Model file for the job. Use its own axes, mm. A direction names the side the tool comes from. Round coordinates to 2 decimals unless told otherwise and drop trailing zeros. Write each loop counter-clockwise with the first axis right and the second up, starting at its lowest first coordinate (ties: lowest second). Pieces come first, ordered by that corner, then holes. Notation, with made-up numbers: (-4, 68) - (9, 68) arc R32 ccw to (9, 100) - close; hole circle Ø11 at (14.25, 23). An arc over 180 degrees is marked (long way). Answer as a JSON object with one key per item and string values. Group by question number.
Autodesk Inventor part; units mm, degrees
ref_plane "YZ Plane" through (0, 0, 0) normal (1, 0, 0) x (0, 1, 0)
ref_plane "XZ Plane" through (0, 0, 0) normal (0, 1, 0) x (-1, 0, 0)
ref_plane "XY Plane" through (0, 0, 0) normal (0, 0, 1) x (1, 0, 0)
sketch "スケッチ1" plane through (0, 0, 0) normal (0, 0, 1) x (1, 0, 0)
  circle A0 centre (1.5, 29.75) radius 0.7835
  circle A1 centre (1.5, 9.75) radius 0.7835
  line L0 (3, 24.75) -> (3, 14.75)
  line L1 (0, 24.75) -> (0, 14.75)
  line L2 (3, 24.75) -> (0, 24.75)
  line L3 (3, 14.75) -> (0, 14.75)
  circle A2 centre (3, 23.65) radius 1.1
  line L4 (3, 19.75) -> (0, 19.75) construction
  line L5 (1.5, 19.75) -> (1.5, 24.75) construction
  circle A3 centre (0, 23.65) radius 1.1
  line L6 (3, 14.75) -> (0, 14.75)
  circle A4 centre (3, 15.85) radius 1.1
  circle A5 centre (0, 15.85) radius 1.1
  circle A6 centre (1.5, 29.75) radius 1.1
  circle A7 centre (1.5, 9.75) radius 1.1
  line L7 (5.9977, 32.75) -> (-2, 32.75) construction
  line L8 (-2, 32.75) -> (-2, 6.75)
  line L9 (-2, 6.75) -> (5.9977, 6.75) construction
  line L10 (5.9977, 6.75) -> (5.9977, 32.75) construction
  line L11 (3, 32.75) -> (0, 32.75)
  line L12 (0, 6.75) -> (3, 6.75)
  circle A8 centre (21.5, 19.75) radius 4
  circle A9 centre (27.5, 19.75) radius 1.1
  circle A10 centre (25.7426, 23.9926) radius 1.1
  circle A11 centre (21.5, 25.75) radius 1.1
  circle A12 centre (17.2574, 23.9926) radius 1.1
  circle A13 centre (15.5, 19.75) radius 1.1
  circle A14 centre (17.2574, 15.5074) radius 1.1
  circle A15 centre (21.5, 13.75) radius 1.1
  circle A16 centre (25.7426, 15.5074) radius 1.1
  circle A17 centre (21.5, 19.75) radius 8
  line L13 (23.1114, 27.586) -> (-2, 32.75)
  line L14 (23.1114, 11.914) -> (-2, 6.75)
  point P0 (0, 0)
  point P1 (1.5, 14.75)
  point P2 (0, 16.95)
  point P3 (0, 22.55)
  point P4 (3, 22.55)
  point P5 (3, 16.95)
  dimension "d0" = 2.2
  dimension "d12" = 16
  dimension "d1" = 2.2
  dimension "d2" = 2
  dimension "d3" = 8
  dimension "d4" = 13
  dimension "d5" = 20
  dimension "d6" = 2.2
  dimension "d7" = 6
  dimension "d10" = 360
extrude "押し出し1" add sketch "スケッチ1" along normal blind 1.5 contours L13 A17 L14 L8 | A17
fillet "フィレット1" radius 2 2 edges at (-2, 32.75, 0.75) (-2, 6.75, 0.75)
sketch "スケッチ2" plane through (0, 0, 0) normal (0, 0, -1) x (-1, 0, 0)
  circle A0 centre (-21.5, 19.75) radius 4
  circle A1 centre (-21.5, 19.75) radius 8
  line L0 (-23.1114, 27.586) -> (-0.4029, 32.2559)
  line L1 (-6.1, 31.0843) -> (-6.1, 8.4157)
  arc A2 (-3, 24.75) -> (-3, 22.55) centre (-3, 23.65) ccw
  line L2 (-0.4029, 7.2441) -> (-23.1114, 11.914)
  circle A3 centre (-21.5, 19.75) radius 10
  line L3 (-14.8725, 27.2384) -> (-6.1, 29.0424)
  line L4 (-6.1, 19.75) -> (-11.5, 19.75) construction
  line L5 (-14.8725, 12.2616) -> (-6.1, 10.4576)
  line L6 (-6.0499, 18.75) -> (-11.5501, 18.75)
  line L7 (-11.5501, 18.75) -> (-11.5501, 20.75)
  line L8 (-11.5501, 20.75) -> (-6.0499, 20.75)
  line L9 (-6.0499, 20.75) -> (-6.0499, 18.75)
  line L10 (-6.0499, 18.75) -> (-11.5501, 20.75) construction
  line L11 (-11.5501, 18.75) -> (-6.0499, 20.75) construction
  point P0 (0, 0)
  point P1 (-4.1, 23.65)
  point P2 (-8.8, 19.75)
  point P3 (-6.1, 18.75)
  point P4 (-6.1, 20.75)
  dimension "d16" = 2
  dimension "d17" = 2
  dimension "d18" = 2
  dimension "d22" = 2
extrude "押し出し2" cut sketch "スケッチ2" against normal blind 1.5 contours L3 L1 L8 A3 | A3 L6 L1 L5
fillet "フィレット2" radius 2 8 edges at (14.8725, 27.2384, 0.75) (14.8725, 12.2616, 0.75) (6.1, 10.4576, 0.75) (6.1, 29.0424, 0.75) (11.5501, 20.75, 0.75) (6.1, 20.75, 0.75) (6.1, 18.75, 0.75) (11.5501, 18.75, 0.75)
equation "\"d18\" = d17"
properties part number "kata_new_1.5" material "アルミニウム 2014-T4"
(1) Drill centre lines: line 1 (X direction, y = 15.5, z = 1.35); line 2 (X direction, y = 23, z = 1.4); line 3 (X direction, y = 22.5, z = 1.1). Where is each one in solid material? Low to high. Write a range as from..to.
(2) Slice it at D-D (x = 15.5). Write the cut outline in (y, z).
(3) Slice it at A-A (x = 21.5). Write the cut outline in (y, z).
(4) Slice it at B-B (y = 19.75). Write the cut outline in (x, z).
(5) Flat gauge pins, fed straight in: pin 1 (2 mm diameter, centred on x = 21.5, y = 13.75, fed in from -Z); pin 2 (0.8 mm diameter, centred on y = 14.5, z = 0.5, fed in from +X); pin 3 (0.8 mm diameter, centred on x = 1.5, z = 0.5, fed in from +Y). Where does each tip first touch, or does it go through?
(6) 3-axis set-ups, long thin cutter, end or side, ignore diameter. For faces 1 (the cylindrical face through (12.288, 15.859, 0.74)), 2 (the cylindrical face through (29.5, 19.9, 0.7)): which of +Z, -Z, +X, -X, +Y, -Y reach the whole face in a straight line?
(7) Slice it at C-C (x = 7). Write the cut outline in (y, z).
(8) Pull direction X, two halves, no side cores. Call faces 3 (the flat face through (10, 20, 1.5)), 4 (the cylindrical face through (-1.1, 23.6, 0.7)), 5 (the flat face through (-2, 20, 1)): pulls with the +X half, pulls with the -X half, needs draft (parallel to the pull), parting line crosses it, or undercut.
Answer:
{
 "1": {"line 1": "-2..-1.04, 4.04..6.1, 12.45..16.16, 18.36..24.64, 26.84..28.28", "line 2": "-2..-0.89, 3.89..6.1, 12.04..16.78, 17.73..19.17, 23.83..25.27, 26.22..28.81", "line 3": "-2..0, 3..6.12, 11.89..18.6, 24.4..29.01"},
 "2": {"outline": "(10.35, 0) - (18.65, 0) - (18.65, 1.5) - (10.35, 1.5) - close; (20.85, 0) - (29.15, 0) - (29.15, 1.5) - (20.85, 1.5) - close"},
 "3": {"outline": "(11.58, 0) - (12.65, 0) - (12.65, 1.5) - (11.58, 1.5) - close; (14.85, 0) - (15.75, 0) - (15.75, 1.5) - (14.85, 1.5) - close; (23.75, 0) - (24.65, 0) - (24.65, 1.5) - (23.75, 1.5) - close; (26.85, 0) - (27.92, 0) - (27.92, 1.5) - (26.85, 1.5) - close"},
 "4": {"outline": "(-2, 0) - (0, 0) - (0, 1.5) - (-2, 1.5) - close; (3, 0) - (14.4, 0) - (14.4, 1.5) - (3, 1.5) - close; (16.6, 0) - (17.5, 0) - (17.5, 1.5) - (16.6, 1.5) - close; (25.5, 0) - (26.4, 0) - (26.4, 1.5) - (25.5, 1.5) - close; (28.6, 0) - (29.5, 0) - (29.5, 1.5) - (28.6, 1.5) - close"},
 "5": {"pin 1": "through", "pin 2": "x = 27.86", "pin 3": "y = 32.11"},
 "6": {"face 1": "+Z, -Z", "face 2": "+Z, -Z, +X"},
 "7": {"outline": "(8.6, 0) - (11.24, 0) - (11.24, 1.5) - (8.6, 1.5) - close; (18.42, 0) - (21.08, 0) - (21.08, 1.5) - (18.42, 1.5) - close; (28.26, 0) - (30.9, 0) - (30.9, 1.5) - (28.26, 1.5) - close"},
 "8": {"face 3": "needs draft", "face 4": "undercut", "face 5": "pulls with the -X half"}
}
